```python
from build123d import *

# Parameters (mm, degrees)
SKETCH1_R           = 10
SKETCH1_R_2         = 8
BOSS_EXTRUDE1_DEPTH = 305
SKETCH2_R           = 10
BOSS_EXTRUDE2_DEPTH = 10
SKETCH3_R           = 6.35
BOSS_EXTRUDE3_DEPTH = 10


with BuildPart() as part:
    # Sketch1 → Boss-Extrude1 (new body)
    with BuildSketch(Plane.XY):
        Circle(SKETCH1_R)
        Circle(SKETCH1_R_2, mode=Mode.SUBTRACT)
    extrude(amount=BOSS_EXTRUDE1_DEPTH)

    # Sketch2 → Boss-Extrude2 (add)
    with BuildSketch(Plane.XY.offset(305)):
        Circle(SKETCH2_R)
    extrude(amount=BOSS_EXTRUDE2_DEPTH)

    # Sketch3 → Boss-Extrude3 (add)
    with BuildSketch(Plane.XY.offset(315)):
        Circle(SKETCH3_R)
    extrude(amount=BOSS_EXTRUDE3_DEPTH)


solid = part.part
```
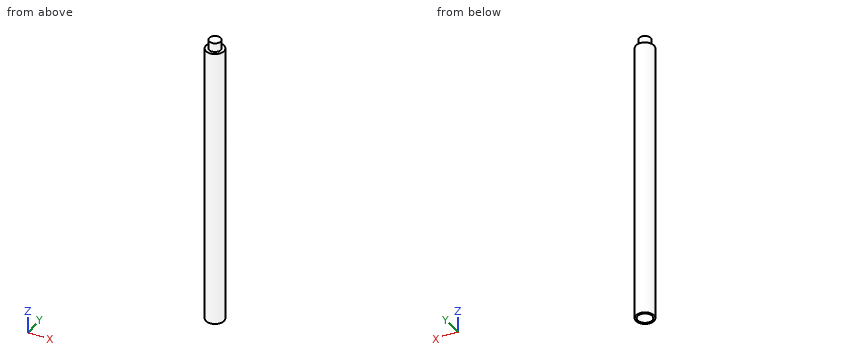
Part model, mm, in its own coordinate system. Give positions to 0.01 mm unless a question says otherwise; leave off trailing zeros. Write each loop counter-clockwise with the first axis right and the second up, starting at its lowest first coordinate (ties: lowest second). Pieces come first, ordered by that corner, then holes. Notation, with made-up numbers: M 80,-18 L 108,-18 A8 ccw 108,-4 Z; hole C 59,27 d9. An arc over 180 degrees is marked long. Use CSV: the item, a comma, the result in double quotes.
Item 1: Pin check, flat tips, straight feed: P1, Ø4, axis at y = -1.5, z = 269.5, coming from the -X side; P2, Ø2, axis at y = -4, z = 128, coming from the -X side; P3, Ø6, axis at x = 7, z = 127, coming from the -Y side; P4, Ø8, axis at x = 0.5, y = -2, coming from the -Z side. Stop position of each tip, or through.
Taken from the geometry:
P1,"stops at x = -10"
P2,"stops at x = -9.54"
P3,"stops at y = -9.17"
P4,"stops at z = 305"
Item 2: Slice it at A-A on x = 0. Write the cut outline in (y, z).
Taken from the geometry:
outline,"M -10,0 L -8,0 L -8,305 L 8,305 L 8,0 L 10,0 L 10,315 L 6.35,315 L 6.35,325 L -6.35,325 L -6.35,315 L -10,315 Z"
Item 3: Drill centre lines: probe 1 along Y at (x, z) = (-0.5, 181.5); probe 2 along Z at (x, y) = (7, 4.25). Where is each one in solid material? Low to high.
Taken from the geometry:
probe 1,"y = -9.99 to -7.98, 7.98 to 9.99"
probe 2,"z = 0 to 315"
Item 4: Slice it at C-C on z = 194.5. Write the cut outline in (x, y).
Taken from the geometry:
outline,"C 0,0 d20; hole C 0,0 d16"
